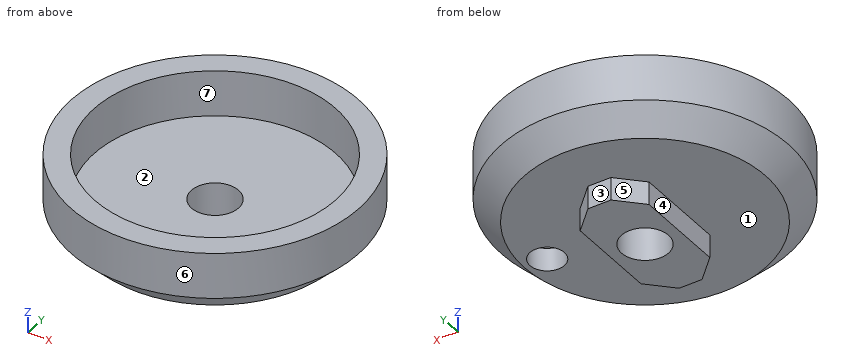
```python
from build123d import *

# Parameters (mm, degrees)
F0_R      = 12.5
F1_DEPTH  = 6
F2_T      = -2
F3_SIZE   = 2
F4_W      = 6
F4_H      = 12
F5_DEPTH  = 2
F6_SIZE   = 2
F7_R      = 2.05
F8_DEPTH  = 25
F9_R      = 1.5
F10_DEPTH = 25


with BuildPart() as f1:
    # F0 (on Top) → F1 (new body)
    with BuildSketch(Plane.XY):
        Circle(F0_R)
    extrude(amount=F1_DEPTH)

    # F2
    f2_openings = [f1.faces().sort_by_distance(p)[0] for p in [
        (0, 0, 6),
    ]]
    offset(amount=F2_T, openings=f2_openings)

    # F3
    f3_edges = [f1.edges().sort_by_distance(p)[0] for p in [
        (-12.5, 0, 0),
    ]]
    chamfer(f3_edges, length=F3_SIZE)

    # F4 (on face) → F5 (join)
    with BuildSketch(Plane(origin=(0, 0, 0), x_dir=(1, 0, 0), z_dir=(0, 0, -1))):
        Rectangle(F4_W, F4_H)
    extrude(amount=F5_DEPTH)

    # F6
    f6_edges = [f1.edges().sort_by_distance(p)[0] for p in [
        (3, -6, -1),
        (-3, -6, -1),
        (3, 6, -1),
        (-3, 6, -1),
    ]]
    chamfer(f6_edges, length=F6_SIZE)

    # F7 (on face) → F8 (cut)
    with BuildSketch(Plane(origin=(0, 0, -2), x_dir=(1, 0, 0), z_dir=(0, 0, -1))):
        Circle(F7_R)
    extrude(amount=-F8_DEPTH, mode=Mode.SUBTRACT)

    # F9 (on face) → F10 (cut)
    with BuildSketch(Plane(origin=(0, 0, 0), x_dir=(1, 0, 0), z_dir=(0, 0, -1))):
        with Locations((8.523585, 0)):
            Circle(F9_R)
    extrude(amount=-F10_DEPTH, mode=Mode.SUBTRACT)


solid = f1.part
```
Model file for the job. Use its own axes, mm. Face numbers are marked on the shaded views. A direction names the side the tool comes from. Give positions to 0.01 mm unless a question says otherwise; leave off trailing zeros. Write each loop counter-clockwise with the first axis right and the second up, starting at its lowest first coordinate (ties: lowest second). Pieces come first, ordered by that corner, then holes. Notation, with made-up numbers: (89.5, -24.75) -> (112.5, -24.75) arc R16 ccw to (112.5, -8.75) -> close; hole circle Ø5 at (51, 3). An arc over 180 degrees is marked (long way). Use CSV: the item, a comma, the result in double quotes. Start each with the question number.
1) Drill centre lines: L1, parallel to Y at x = 0, z = -0.65; L2, parallel to Y at x = 0, z = 5; L3, parallel to X at y = 0, z = -0.55. Where is each one in solid material? Low to high.
2) Cut at A-A on y = 0. List the corners of the cut face in (x, z), plus the area to 3 significant figures.
3) Cut at B-B on x = 0. List the corners of the cut face in (y, z).
4) Pin check, flat tips, straight feed: P1, Ø1.5, axis at y = -5.5, z = 0.5, coming from the -X side; P2, Ø5, axis at x = 8.52, y = 0, coming from the -Z side; P3, Ø1.6, axis at x = -0.5, z = -1.5, coming from the +Y side. Stop position of each tip, or through.
5) Tool access for the marked faces 4, 5, 6 and 7: list every direction of +Z, -Z, +X, -X, +Y, -Y with a clear straight run to the whole face (end or side of a thin tool).
6) Two-plate mould, pull along Y, no slides. Class the marked faces 1, 2 and 3: released by +Y, released by -Y, zero draft, split by the parting line, or undercut.
7) Cut at C-C on z = 4.25. List the corners of the cut face in (x, y), plus the area to 3 significant figures.
Final values:
1,L1,"y = -6 to -2.05, 2.05 to 6"
1,L2,"y = -12.5 to -10.5, 10.5 to 12.5"
1,L3,"x = -3 to -2.05, 2.05 to 3"
2,outline,"(-12.5, 2) -> (-10.5, 0) -> (-3, 0) -> (-3, -2) -> (-2.05, -2) -> (-2.05, 2) -> (-10.5, 2) -> (-10.5, 6) -> (-12.5, 6) -> close; (2.05, -2) -> (3, -2) -> (3, 0) -> (7.02, 0) -> (7.02, 2) -> (2.05, 2) -> close; (10.02, 0) -> (10.5, 0) -> (12.5, 2) -> (12.5, 6) -> (10.5, 6) -> (10.5, 2) -> (10.02, 2) -> close"
2,area,"51.6 mm2"
3,outline,"(-12.5, 2) -> (-10.5, 0) -> (-6, 0) -> (-6, -2) -> (-2.05, -2) -> (-2.05, 2) -> (-10.5, 2) -> (-10.5, 6) -> (-12.5, 6) -> close; (2.05, -2) -> (6, -2) -> (6, 0) -> (10.5, 0) -> (12.5, 2) -> (12.5, 6) -> (10.5, 6) -> (10.5, 2) -> (2.05, 2) -> close"
4,P1,"stops at x = -10.47"
4,P2,"stops at z = 0"
4,P3,"stops at y = 6"
5,face 4,"-Z, -X, +Y, -Y"
5,face 5,"-Z, -X, +Y"
5,face 6,"+Z, -Z"
5,face 7,"+Z"
6,face 1,"zero draft"
6,face 2,"undercut"
6,face 3,"released by +Y"
7,outline,"circle Ø25 at (0, 0); hole circle Ø21 at (0, 0)"
7,area,"145 mm2"
